```python
from build123d import *

# Parameters (mm, degrees)
EXTRUDE_1_DEPTH     = 8
SKETCH_2_W          = 7
SKETCH_2_H          = 60
EXTRUDE_2_DEPTH     = 22
MM_1_D              = 9
HOLE_WIZARD_M5_1_D  = 4.2
SKETCH_5_R          = 11
CUT_EXTRUDE_1_DEPTH = 10


with BuildPart() as part:
    # 草图1 → 凸台-拉伸1 (new body)
    with BuildSketch(Plane(origin=(0, 0, 0), x_dir=(1, 0, 0), z_dir=(0, 1, 0))):
        with BuildLine():
            Line((-14.75, 30), (40.25, 30))
            Line((40.25, 30), (40.25, -30))
            Line((40.25, -30), (-14.75, -30))
            ThreePointArc((-14.75, -30), (-44.75, 0), (-14.75, 30))
        make_face()
    extrude(amount=EXTRUDE_1_DEPTH)

    # 草图2 → 凸台-拉伸2 (add)
    with BuildSketch(Plane(origin=(0, 8, 0), x_dir=(1, 0, 0), z_dir=(0, 1, 0))):
        with Locations((36.75, 0)):
            Rectangle(SKETCH_2_W, SKETCH_2_H)
    extrude(amount=EXTRUDE_2_DEPTH)

    # 大小mm 暗销孔1 (through all)
    with Locations(Plane(origin=(40.25, 15, 15), x_dir=(0, 0, 1), z_dir=(1, 0, 0))):
        with Locations((0, 0), (-30, 0)):
            Hole(MM_1_D / 2)

    # M5 螺纹孔1 (through all)
    with Locations(Plane(origin=(-31.75, 0, 15), x_dir=(0, 0, -1), z_dir=(0, -1, 0))):
        with Locations((0, 0), (0, 50), (30, 50), (30, 0)):
            Hole(HOLE_WIZARD_M5_1_D / 2)

    # 草图5 → 切除-拉伸1 (cut)
    with BuildSketch(Plane.XZ):
        with Locations((-6.75, 0)):
            Circle(SKETCH_5_R)
    extrude(amount=-CUT_EXTRUDE_1_DEPTH, mode=Mode.SUBTRACT)


solid = part.part
```
Part model, mm, in its own coordinate system. A direction names the side the tool comes from. Coordinates: 2 decimals unless noted, no trailing zeros. Loops run counter-clockwise (first coordinate to the right, second up) from the corner with the lowest first, then second, coordinate; pieces in that order, holes last. Notation, with made-up numbers: (40, 82.25) - (56, 82.25) arc R12 ccw to (56, 100.25) - close; hole circle Ø6 at (62.5, -22). An arc over 180 degrees is marked (long way). Write item = value, one per line. Start each with the question number.
Item 1: Cut at A-A, the plane x = 18.25. Give the cut face in (y, z), and give its area (3 significant figures).
Item 2: Cut at D-D, the plane x = -31.75. Give the cut face in (y, z).
Item 3: Flat gauge pins, fed straight in: pin 1 Ø5.5 at (x, z) = (18.25, -15) entering from +Y; pin 2 Ø1 at (y, z) = (19.5, -1.5) entering from -X; pin 3 Ø5 at (y, z) = (9.5, -9.5) entering from -X. Where does each tip first touch, or does it go through?
Item 4: 3-axis set-ups, long thin cutter, end or side, ignore diameter. For faces 5 (the flat face through (40.25, 15, 0)), 6 (the flat face through (33.25, 19, 0)): which of +Z, -Z, +X, -X, +Y, -Y reach the whole face in a straight line?
Item 5: Mould opens along Y. For faces 1 (the cylindrical face through (36.7, 11.96, 18.32)), 2 (the cylindrical face through (-9.13, 3.94, -10.74)), 3 (the flat face through (37, 30, 0)), 4 (the cylindrical face through (36.7, 10.54, -14.41)) say: released by +Y, released by -Y, zero draft, split by the parting line, or undercut.
Item 6: Cut at C-C, the plane x = -6.75. Give the cut face in (y, z), and give its area (3 significant figures).
Item 7: Wall check: L1, parallel to X at y = 4.5, z = -15; L2, parallel to Z at x = -3.5, y = 3.75; L3, parallel to Y at x = 27, z = 16. Give the ranges that are in metal, low to high. Write a range as from..to.
Item 8: Cut at B-B, the plane z = 15. Give the cut face in (x, y), and give its area (3 significant figures).
The answers:
q1.outline = (0, -30) - (8, -30) - (8, -17.1) - (0, -17.1) - close; (0, -12.9) - (8, -12.9) - (8, 12.9) - (0, 12.9) - close; (0, 17.1) - (8, 17.1) - (8, 30) - (0, 30) - close
q1.area = 413 mm2
q2.outline = (0, -24.72) - (8, -24.72) - (8, -17.1) - (0, -17.1) - close; (0, -12.9) - (8, -12.9) - (8, 12.9) - (0, 12.9) - close; (0, 17.1) - (8, 17.1) - (8, 24.72) - (0, 24.72) - close
q3.pin_1 = 8
q3.pin_2 = 33.25
q3.pin_3 = -43.8
q4.face_5 = +Z, -Z, +X, +Y, -Y
q4.face_6 = +Z, -Z, -X, +Y
q5.face_1 = undercut
q5.face_2 = zero draft
q5.face_3 = released by +Y
q5.face_4 = undercut
q6.outline = (0, -30) - (8, -30) - (8, -11) - (0, -11) - close; (0, 11) - (8, 11) - (8, 30) - (0, 30) - close
q6.area = 304 mm2
q7.L1 = -40.73..-33.85, -29.65..16.15, 20.35..40.25
q7.L2 = -30..-10.51, 10.51..30
q7.L3 = 0..8
q8.outline = (-40.73, 0) - (-33.85, 0) - (-33.85, 8) - (-40.73, 8) - close; (-29.65, 0) - (16.15, 0) - (16.15, 8) - (-29.65, 8) - close; (20.35, 0) - (40.25, 0) - (40.25, 10.5) - (33.25, 10.5) - (33.25, 8) - (20.35, 8) - close; (33.25, 19.5) - (40.25, 19.5) - (40.25, 30) - (33.25, 30) - close
q8.area = 672 mm2
